from build123d import *

# Parameters (mm, degrees)
SKETCH1_R           = 25
BOSS_EXTRUDE1_DEPTH = 600
SKETCH1_3_R         = 40
SKETCH1_3_R_2       = 25
BOSS_EXTRUDE2_DEPTH = 50
BOSS_EXTRUDE3_DEPTH = 20
SKETCH30_W          = 5.156865167
SKETCH30_H          = 15
CHAMFER1_SIZE       = 1
SKETCH31_W          = 59.59
SKETCH31_H          = 7
BOSS_EXTRUDE4_DEPTH = 557
SKETCH32_W          = 21
SKETCH32_H          = 8.16254176
CUT_EXTRUDE1_DEPTH  = 570
SHELL2_DEPTH        = 596
SHELL2_2_OUTLINE_R  = 36
SHELL2_2_DEPTH      = 46
SHELL2_START        = 596
SHELL2_3_DEPTH      = 20


# Read off the part's stored shape, not the designer's step: Shell2
with BuildPart() as part:
    # Sketch1 → Boss-Extrude1 (new body)
    with BuildSketch(Plane(origin=(0, 0, 0), x_dir=(1, 0, 0), z_dir=(0, 1, 0))):
        with Locations(Location((0, 0, 0), (0, 0, 270))):
            Circle(SKETCH1_R)
    extrude(amount=BOSS_EXTRUDE1_DEPTH)

    # Sketch1<3> → Boss-Extrude2 (add)
    with BuildSketch(Plane(origin=(0, 0, 0), x_dir=(1, 0, 0), z_dir=(0, 1, 0))):
        with Locations(Location((0, 0, 0), (0, 0, 270))):
            Circle(SKETCH1_3_R)
        with Locations(Location((0, 0, 0), (0, 0, 270))):
            Circle(SKETCH1_3_R_2, mode=Mode.SUBTRACT)
    extrude(amount=BOSS_EXTRUDE2_DEPTH)

    # Sketch2 → Boss-Extrude3 (add)
    with BuildSketch(Plane(origin=(0, 600, 0), x_dir=(1, 0, 0), z_dir=(0, 1, 0))):
        with BuildLine():
            Line((19.843134833, 2.5), (23.869436525, 2.5))
            ThreePointArc((23.869436525, 2.5), (24, 0), (23.869436525, -2.5))
            Line((23.869436525, -2.5), (19.843134833, -2.5))
            ThreePointArc((19.843134833, -2.5), (0, -20), (-19.843134833, -2.5))
            Line((-19.843134833, -2.5), (-23.869436525, -2.5))
            ThreePointArc((-23.869436525, -2.5), (-24, 0), (-23.869436525, 2.5))
            Line((-23.869436525, 2.5), (-19.843134833, 2.5))
            ThreePointArc((-19.843134833, 2.5), (0, 20), (19.843134833, 2.5))
        make_face()
    extrude(amount=BOSS_EXTRUDE3_DEPTH)

    # Sketch30 → Cut-Revolve1 (revolve, cut)
    with BuildSketch(Plane.XY, mode=Mode.PRIVATE) as cut_revolve1_sk:
        with Locations((22.421567417, 607.5)):
            Rectangle(SKETCH30_W, SKETCH30_H)
    revolve(cut_revolve1_sk.sketch.rotate(Axis((0, 498.152783653, 0), (0, 1, 0)), 90), axis=Axis((0, 498.152783653, 0), (0, 1, 0)), mode=Mode.SUBTRACT)

    # Chamfer1
    chamfer1_edges = [part.edges().sort_by_distance(p)[0] for p in [
        (-24, 620, 0),
        (24, 620, 0),
        (-24, 615, 0),
        (24, 615, 0),
    ]]
    chamfer(chamfer1_edges, length=CHAMFER1_SIZE)

    # Sketch31 → Boss-Extrude4 (add)
    with BuildSketch(Plane(origin=(0, 600, 0), x_dir=(1, 0, 0), z_dir=(0, 1, 0))):
        Rectangle(SKETCH31_W, SKETCH31_H)
    extrude(amount=-BOSS_EXTRUDE4_DEPTH)

    # Sketch32 → Cut-Extrude1 (cut)
    with BuildSketch(Plane(origin=(0, 620, 0), x_dir=(1, 0, 0), z_dir=(0, 1, 0))):
        with Locations((0, -20.91872912)):
            Rectangle(SKETCH32_W, SKETCH32_H)
    extrude(amount=-CUT_EXTRUDE1_DEPTH, mode=Mode.SUBTRACT)

    # Shell2 outline → Shell2 (cut)
    with BuildSketch(Plane(origin=(0, 0, 0), x_dir=(1, 0, 0), z_dir=(0, 1, 0))):
        with BuildLine():
            ThreePointArc((14.5, -15.190457531), (0, 21), (-14.5, -15.190457531))
            Line((-14.5, -15.190457531), (-14.5, -12.83745824))
            Line((-14.5, -12.83745824), (14.5, -12.83745824))
            Line((14.5, -12.83745824), (14.5, -15.190457531))
        make_face()
    extrude(amount=SHELL2_DEPTH, mode=Mode.SUBTRACT)

    # Shell2 2 outline → Shell2 2 (cut)
    with BuildSketch(Plane(origin=(0, 0, 0), x_dir=(1, 0, 0), z_dir=(0, 1, 0))):
        Circle(SHELL2_2_OUTLINE_R)
        with BuildLine():
            Line((-14.5, -12.83745824), (-14.5, -15.190457531))
            ThreePointArc((-14.5, -15.190457531), (0, 21), (14.5, -15.190457531))
            Line((14.5, -15.190457531), (14.5, -12.83745824))
            Line((14.5, -12.83745824), (-14.5, -12.83745824))
        make_face(mode=Mode.SUBTRACT)
    extrude(amount=SHELL2_2_DEPTH, mode=Mode.SUBTRACT)

    # Shell2 3 outline → Shell2 3 (cut)
    with BuildSketch(Plane(origin=(0, 0, 0), x_dir=(1, 0, 0), z_dir=(0, 1, 0)).offset(SHELL2_START)):
        with BuildLine():
            ThreePointArc((9.284642549, -12.83745824), (0, 15.843134833), (-9.284642549, -12.83745824))
            Line((-9.284642549, -12.83745824), (9.284642549, -12.83745824))
        make_face()
    extrude(amount=SHELL2_3_DEPTH, mode=Mode.SUBTRACT)


solid = part.part
Verification items for the finished model (mm, model axes). A direction names the side the tool comes from. Give positions to 0.01 mm unless a question says otherwise; leave off trailing zeros. Order: outer loops, then holes, each group sorted by start corner. A loop starts at its lowest first (then second) coordinate and runs counter-clockwise, first axis right, second up. Notation, with made-up numbers: M 16,-28 L 43,-28 A15 ccw 43,-17 Z; hole C 67,-22.5 d7. An arc over 180 degrees is marked long. Answer as a JSON object with one key per item and string values. Group by question number.
1) Mould release check, pull along Z, two halves, no side actions. Record for faces 5 (the face through (0.72, 607.6, -19.83)), 6 (the face through (-4.686, 22.678, -35.694)), 7 (the face through (-21, 615, -2)): released by +Z, released by -Z, zero draft, split by the parting line, or undercut.
2) Cross-section at A-A (y = 112). Enter the section's corners in (x, z) (3 decimals).
3) Depth check by flat-ended pin: pin 1 Ø3 at (x, z) = (-10, 5.5) entering from -Y; pin 2 Ø1.5 at (x, y) = (-16.5, 260) entering from -Z; pin 3 Ø5 at (y, z) = (98, -9) entering from -X. Enter the tip coordinate at first touch or a pass-through.
4) Scan lines: line 1 along X through (y, z) = (275, 0) (3 decimals); line 2 along X through (y, z) = (11, 0); line 3 along Z through (x, y) = (0, 611.5). Record each from-to range of solid material in increasing order. Write a range as [from, to].
5) Access from +Z, -Z, +X, -X, +Y, -Y to the whole of each face (thin tool, end or side, straight path). Record for faces 1 (the face through (0, 339, 16.837)), 2 (the face through (0, 617, -20)), 3 (the face through (20, 321, 15)), 4 (the face through (0, 327, 12.837)).
6) Cross-section at B-B (x = 0). Enter the section's corners in (y, z).
Result sheet:
{
 "1": {"face 5": "split by the parting line", "face 6": "undercut", "face 7": "zero draft"},
 "2": {"outline": "M -29.795,-3.5 L -24.754,-3.5 A25 ccw 24.754,-3.5 L 29.795,-3.5 L 29.795,3.5 L 24.754,3.5 A25 ccw 10.5,22.688 L 10.5,16.837 L -10.5,16.837 L -10.5,22.688 A25 ccw -24.754,3.5 L -29.795,3.5 Z; hole M -14.5,12.837 L -14.5,15.19 A21 ccw long 14.5,15.19 L 14.5,12.837 Z"},
 "3": {"pin 1": "stops at y = 616", "pin 2": "stops at z = -19.41", "pin 3": "stops at x = -24.14"},
 "4": {"line 1": "x = [-29.795, -21], [21, 29.795]", "line 2": "x = [-40, -36], [36, 40]", "line 3": "z = [-19.84, -15.84], [12.84, 16.84]"},
 "5": {"face 1": "+Z, +Y", "face 2": "-Z, +Y", "face 3": "+Z, +X, +Y", "face 4": "-Y"},
 "6": {"outline": "M 0,-40 L 50,-40 L 50,-25 L 600,-25 L 600,-19.84 L 615,-19.84 L 615,-20 L 620,-20 L 620,16.84 L 50,16.84 L 50,40 L 0,40 L 0,36 L 46,36 L 46,12.84 L 616,12.84 L 616,-15.84 L 596,-15.84 L 596,-21 L 46,-21 L 46,-36 L 0,-36 Z"}
}
